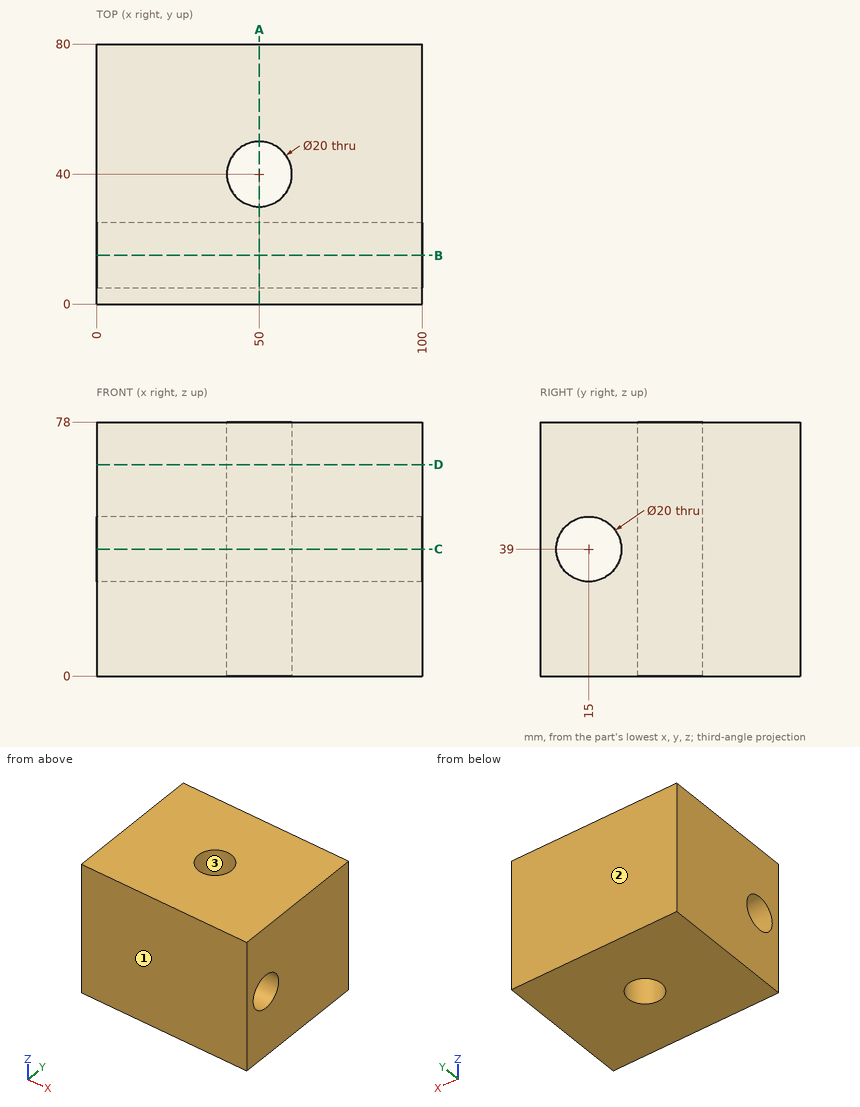
The figure shows three views and two pictorial views of one solid part (mm, origin at its lowest corner). Answer the questions. Coordinates: 2 decimals unless noted, no trailing zeros. Write each loop counter-clockwise with the first axis right and the second up, starting at its lowest first coordinate (ties: lowest second). Pieces come first, ordered by that corner, then holes. Notation, with made-up numbers: (-8, -33.75) -> (-4, -33.75) arc R25 ccw to (-4, -15.75) -> close; hole circle Ø4 at (44.5, -30). An arc over 180 degrees is marked (long way). Return JSON: item names as keys, results as strings.
1. A cutting plane is placed at C-C (z = 39). Determine the outline of the cut face in (x, y), and give its area (3 significant figures).
Found:
{"outline": "(0, 0) -> (100, 0) -> (100, 5) -> (0, 5) -> close; (0, 25) -> (100, 25) -> (100, 80) -> (0, 80) -> close; hole circle Ø20 at (50, 40)", "area": "5,690 mm2"}
2. A cutting plane is placed at A-A (x = 50). Determine the outline of the cut face in (y, z), and give its area (3 significant figures).
Found:
{"outline": "(0, 0) -> (30, 0) -> (30, 78) -> (0, 78) -> close; (50, 0) -> (80, 0) -> (80, 78) -> (50, 78) -> close; hole circle Ø20 at (15, 39)", "area": "4,370 mm2"}
3. A cutting plane is placed at D-D (z = 65). Determine the outline of the cut face in (x, y), and give its area (3 significant figures).
Found:
{"outline": "(0, 0) -> (100, 0) -> (100, 80) -> (0, 80) -> close; hole circle Ø20 at (50, 40)", "area": "7,690 mm2"}
4. Find the intervals of material crossed by line 1 along Z through (x, y) = (36.5, 15); line 2 along Z through (x, y) = (22, 22); line 3 along Y through (x, z) = (50.5, 14.5), in increasing order. Write a range as from..to.
Found:
{"line 1": "0..29, 49..78", "line 2": "0..31.86, 46.14..78", "line 3": "0..30.01, 49.99..80"}
5. Determine the mould class of the marked faces 1, 2 and 3 for opening direction Y: pulls with the +Y half, pulls with the -Y half, needs draft (parallel to the pull), parting line crosses it, or undercut.
Found:
{"face 1": "pulls with the -Y half", "face 2": "pulls with the +Y half", "face 3": "undercut"}
6. A cutting plane is placed at B-B (y = 15). Determine the outline of the cut face in (x, z).
Found:
{"outline": "(0, 0) -> (100, 0) -> (100, 29) -> (0, 29) -> close; (0, 49) -> (100, 49) -> (100, 78) -> (0, 78) -> close"}
